Part model, mm, in its own coordinate system. Face numbers are marked on the shaded views. A direction names the side the tool comes from. Round coordinates to 2 decimals unless told otherwise and drop trailing zeros. Write each loop counter-clockwise with the first axis right and the second up, starting at its lowest first coordinate (ties: lowest second). Pieces come first, ordered by that corner, then holes.
1) Saw through at A-A on z = -36. Write the cut outline in (x, y).
2) Flat gauge pins, fed straight in: pin 1 (1.5 mm diameter, centred on x = 8.5, y = 4.5, fed in from +Z); pin 2 (3 mm diameter, centred on x = -33.5, y = -1, fed in from +Z); pin 3 (6 mm diameter, centred on x = -25, y = 3.5, fed in from +Z). Where does each tip first touch, or does it go through?
3) Drill centre lines: L1, parallel to X at y = -3, z = 0; L2, parallel to X at y = 4.5, z = 30; L3, parallel to X at y = 0.85, z = 0. Where is each one in solid material? Low to high.
4) Which spindle directions (+Z, -Z, +X, -X, +Y, -Y) get a long thin tool onto all of the face, cutting with end or side? Do the marked faces 3 and 4. Say none if no direction does.
5) Pull direction X, two halves, no side cores. Call the marked faces 1 and 2: +X half, -X half, draft (parallel to the pull), parting line (faces both ways), or undercut.
6) Saw through at B-B on x = -34. Write the cut outline in (y, z), and give its area (3 significant figures).
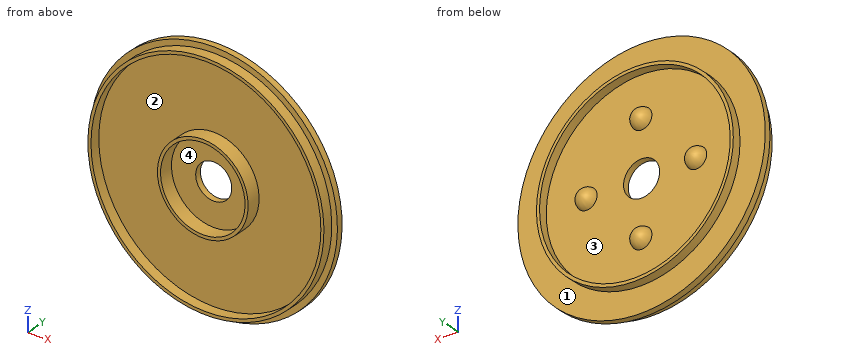
```python
from build123d import *

# Parameters (mm, degrees)
SKETCH3_R           = 60
SKETCH3_R_2         = 8.75
BOSS_EXTRUDE1_DEPTH = 3
SKETCH4_R           = 57.25
SKETCH4_R_2         = 55.75
BOSS_EXTRUDE2_DEPTH = 5
SKETCH5_R           = 22
SKETCH5_R_2         = 20.5
BOSS_EXTRUDE3_DEPTH = 7
SKETCH6_R           = 47.75
SKETCH6_R_2         = 46.25
BOSS_EXTRUDE4_DEPTH = 4.3
SKETCH10_R          = 5
BOSS_EXTRUDE5_DEPTH = 4.3
FILLET2_R           = 5


with BuildPart() as part:
    # Sketch3 → Boss-Extrude1 (new body)
    with BuildSketch(Plane(origin=(0, 0, 0), x_dir=(1, 0, 0), z_dir=(0, 1, 0))):
        with Locations(Location((0, 0, 0), (0, 0, 270))):
            Circle(SKETCH3_R)
        with Locations(Location((0, 0, 0), (0, 0, 270))):
            Circle(SKETCH3_R_2, mode=Mode.SUBTRACT)
    extrude(amount=BOSS_EXTRUDE1_DEPTH)

    # Sketch4 → Boss-Extrude2 (add)
    with BuildSketch(Plane.XZ):
        with Locations(Location((0, 0, 0), (0, 0, 90))):
            Circle(SKETCH4_R)
        with Locations(Location((0, 0, 0), (0, 0, 270))):
            Circle(SKETCH4_R_2, mode=Mode.SUBTRACT)
    extrude(amount=BOSS_EXTRUDE2_DEPTH)

    # Sketch5 → Boss-Extrude3 (add)
    with BuildSketch(Plane.XZ):
        with Locations(Location((0, 0, 0), (0, 0, 90))):
            Circle(SKETCH5_R)
        with Locations(Location((0, 0, 0), (0, 0, 270))):
            Circle(SKETCH5_R_2, mode=Mode.SUBTRACT)
    extrude(amount=BOSS_EXTRUDE3_DEPTH)

    # Sketch6 → Boss-Extrude4 (add)
    with BuildSketch(Plane(origin=(0, 3, 0), x_dir=(1, 0, 0), z_dir=(0, 1, 0))):
        with Locations(Location((0, 0, 0), (0, 0, 90))):
            Circle(SKETCH6_R)
        with Locations(Location((0, 0, 0), (0, 0, 90))):
            Circle(SKETCH6_R_2, mode=Mode.SUBTRACT)
    extrude(amount=BOSS_EXTRUDE4_DEPTH)

    # Sketch10 → Boss-Extrude5 (add)
    with BuildSketch(Plane(origin=(0, 3, 0), x_dir=(1, 0, 0), z_dir=(0, 1, 0))):
        with Locations(Location((0, 26.574961269, 0), (0, 0, 270))):
            Circle(SKETCH10_R)
        with Locations(Location((26.574961269, 0, 0), (0, 0, 270))):
            Circle(SKETCH10_R)
        with Locations(Location((0, -26.574961269, 0), (0, 0, 270))):
            Circle(SKETCH10_R)
        with Locations(Location((-26.574961269, 0, 0), (0, 0, 270))):
            Circle(SKETCH10_R)
    extrude(amount=BOSS_EXTRUDE5_DEPTH)

    # Fillet2
    # the kernel refuses this fillet: 5 mm, written as the material it takes off along each edge
    with BuildSketch(Plane(origin=(0, 7.3, -26.574961269), x_dir=(0, 0, 1), z_dir=(-1, 0, 0))) as fillet2_piece_1:
        with BuildLine():
            CenterArc((0.049242482, -5), FILLET2_R, 8.047846247, 81.952153753)
            Line((0.049242482, 0), (0.049242482, 0.1))
            Line((0.049242482, 0.1), (5, 0.1))
            Line((5, 0.1), (5.1, 0))
            ThreePointArc((5.1, 0), (5.1, -2.15), (5.09901515, -4.286))
            Line((5.09901515, -4.286), (5, -4.3))
        make_face()
    revolve(axis=Axis((0, 7.3, -26.574961269), (0, 1, 0)), mode=Mode.SUBTRACT)
    with BuildSketch(Plane(origin=(26.574961269, 7.3, 0), x_dir=(0, 0, 1), z_dir=(-1, 0, 0))) as fillet2_piece_2:
        with BuildLine():
            CenterArc((0.049242482, -5), FILLET2_R, 8.047846247, 81.952153753)
            Line((0.049242482, 0), (0.049242482, 0.1))
            Line((0.049242482, 0.1), (5, 0.1))
            Line((5, 0.1), (5.1, 0))
            ThreePointArc((5.1, 0), (5.1, -2.15), (5.09901515, -4.286))
            Line((5.09901515, -4.286), (5, -4.3))
        make_face()
    revolve(axis=Axis((26.574961269, 7.3, 0), (0, 1, 0)), mode=Mode.SUBTRACT)
    with BuildSketch(Plane(origin=(0, 7.3, 26.574961269), x_dir=(0, 0, 1), z_dir=(-1, 0, 0))) as fillet2_piece_3:
        with BuildLine():
            CenterArc((0.049242482, -5), FILLET2_R, 8.047846247, 81.952153753)
            Line((0.049242482, 0), (0.049242482, 0.1))
            Line((0.049242482, 0.1), (5, 0.1))
            Line((5, 0.1), (5.1, 0))
            ThreePointArc((5.1, 0), (5.1, -2.15), (5.09901515, -4.286))
            Line((5.09901515, -4.286), (5, -4.3))
        make_face()
    revolve(axis=Axis((0, 7.3, 26.574961269), (0, 1, 0)), mode=Mode.SUBTRACT)
    with BuildSketch(Plane(origin=(-26.574961269, 7.3, 0), x_dir=(0, 0, 1), z_dir=(-1, 0, 0))) as fillet2_piece_4:
        with BuildLine():
            CenterArc((0.049242482, -5), FILLET2_R, 8.047846247, 81.952153753)
            Line((0.049242482, 0), (0.049242482, 0.1))
            Line((0.049242482, 0.1), (5, 0.1))
            Line((5, 0.1), (5.1, 0))
            ThreePointArc((5.1, 0), (5.1, -2.15), (5.09901515, -4.286))
            Line((5.09901515, -4.286), (5, -4.3))
        make_face()
    revolve(axis=Axis((-26.574961269, 7.3, 0), (0, 1, 0)), mode=Mode.SUBTRACT)


solid = part.part
```
Completed:
1. outline: (-48, 0) - (-44.51, 0) - (-44.51, -5) - (-42.57, -5) - (-42.57, 0) - (42.57, 0) - (42.57, -5) - (44.51, -5) - (44.51, 0) - (48, 0) - (48, 3) - (31.37, 3) - (31.37, 7.3) - (29.04, 7.3) - (29.04, 3) - (-29.04, 3) - (-29.04, 7.3) - (-31.37, 7.3) - (-31.37, 3) - (-48, 3) - close
2. pin 1: stops at z = 47.12
2. pin 2: stops at z = 50.51
2. pin 3: stops at z = 55.8
3. L1: x = -57.25 to -55.75, -22 to -20.5, 20.5 to 22, 55.75 to 57.25
3. L2: x = -37.15 to -35.2, -2.98 to 2.98, 35.2 to 37.15
3. L3: x = -60 to -8.75, 8.75 to 60
4. face 3: +Y
4. face 4: -Y
5. face 1: draft
5. face 2: undercut
6. outline: (-5, -46.06) - (0, -46.06) - (0, -49.44) - (3, -49.44) - (3, -33.53) - (7.3, -33.53) - (7.3, -31.35) - (3, -31.35) - (3, 31.35) - (7.3, 31.35) - (7.3, 33.53) - (3, 33.53) - (3, 49.44) - (0, 49.44) - (0, 46.06) - (-5, 46.06) - (-5, 44.18) - (0, 44.18) - (0, -44.18) - (-5, -44.18) - close
6. area: 334 mm2
